Can you work these out from the drawing? Everything is in mm from the part's minimum corner. A direction names the side the tool comes from. Give positions to 0.01 mm unless a question says otherwise; leave off trailing zeros. Loops run counter-clockwise (first coordinate to the right, second up) from the corner with the lowest first, then second, coordinate; pieces in that order, holes last. Notation, with made-up numbers: M -34.75,64.25 L -30.75,64.25 A17 cw -30.75,69.25 Z; hole C -27,82.5 d1. An arc over 180 degrees is marked long. Use CSV: the item, a comma, the result in double quotes.
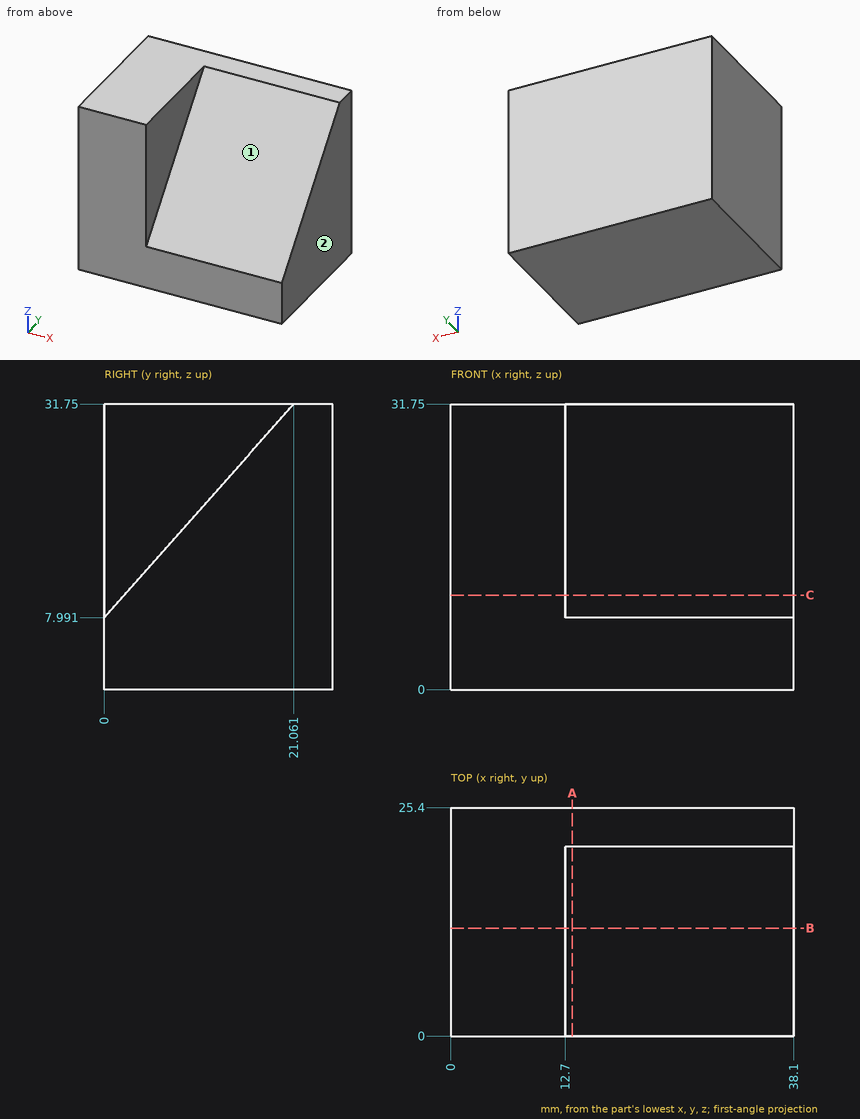
Q1. I want a section at A-A, the plane x = 13.5. Please give me the cut outline in (y, z).
Model answer:
outline,"M 0,0 L 25.4,0 L 25.4,31.75 L 21.06,31.75 L 0,7.99 Z"
Q2. I'm going to push flat-ended pins straight in: P1, Ø4, axis at x = 16, z = 13.5, coming from the -Y side; P2, Ø1, axis at x = 34, y = 18, coming from the +Z side. Where does each tip first touch, or does it pass through?
Model answer:
P1,"y = 3.11"
P2,"z = 28.86"
Q3. For the marked faces 1 and 2, which set-ups out of +Z, -Z, +X, -X, +Y, -Y let a thin tool reach every point of the face, with its end or its side?
Model answer:
face 1,"+Z, +X, -Y"
face 2,"+Z, -Z, +X, +Y, -Y"
Q4. I want a section at C-C, the plane z = 10.5. Please give me the cut outline in (x, y) (1 decimal).
Model answer:
outline,"M 0,0 L 12.7,0 L 12.7,2.2 L 38.1,2.2 L 38.1,25.4 L 0,25.4 Z"
Q5. Please list where these lines run through material, in increasing order: L1, parallel to X at y = 15.75, z = 30; L2, parallel to Z at x = 18.5, y = 10; L3, parallel to Z at x = 25.5, y = 7.75 (1 decimal). Write a range as from..to.
Model answer:
L1,"0..12.7"
L2,"0..19.27"
L3,"0..16.7"
Q6. I want a section at B-B, the plane y = 12. Please give me the cut outline in (x, z), then the cut area to 3 significant figures.
Model answer:
outline,"M 0,0 L 38.1,0 L 38.1,21.53 L 12.7,21.53 L 12.7,31.75 L 0,31.75 Z"
area,"950 mm2"
